```python
from build123d import *

# Parameters (mm, degrees)
CROQUIS1_W                       = 1396
CROQUIS1_H                       = 387.3
BRIDA_BASE1_DEPTH                = 3.175
TALADRO_DE_MARGEN_PARA_M51_D     = 5.5
BRIDA_DE_ARISTA1_STRIP_W         = 32.7
BRIDA_DE_ARISTA1_STRIP_H         = 3.175
BRIDA_DE_ARISTA1_STRIP_CUT_DEPTH = 1396
BRIDA_DE_ARISTA1_DEPTH           = 1396
TALADRO_DE_MARGEN_PARA_M52_D     = 5.5


# Sheet-metal steps are written as plain solids
with BuildPart() as part:
    # Croquis1 → Brida base1 (new body)
    with BuildSketch(Plane(origin=(0, 0, 0), x_dir=(1, 0, 0), z_dir=(0, 1, 0))):
        with Locations((-11.780590717, 234.868987342)):
            Rectangle(CROQUIS1_W, CROQUIS1_H)
    extrude(amount=-BRIDA_BASE1_DEPTH)

    # Taladro de margen para M51 (through all)
    with Locations(Plane(origin=(0, -3.175, 0), x_dir=(-1, 0, 0), z_dir=(0, -1, 0))):
        with Locations((508.430590717, 166.618987342), (508.430590717, 341.218987342), (308.430590717, 166.618987342), (308.430590717, 341.218987342), (108.430590717, 166.618987342), (108.430590717, 341.218987342), (-91.569409283, 166.618987342), (-91.569409283, 341.218987342), (-291.569409283, 166.618987342), (-291.569409283, 341.218987342), (-491.569409283, 166.618987342), (-491.569409283, 341.218987342), (667.430590717, 166.618987342), (667.430590717, 341.218987342), (-650.569409283, 166.618987342), (-650.569409283, 341.218987342)):
            Hole(TALADRO_DE_MARGEN_PARA_M51_D / 2)

    # Brida de arista1 strip (across the edge) → Brida de arista1 strip cut (cut)
    with BuildSketch(Plane(origin=(-709.780590717, -3.175, -428.518987342), x_dir=(0, 0, 1), z_dir=(1, 0, 0))):
        with Locations((-3.175, -1.5875)):
            Rectangle(BRIDA_DE_ARISTA1_STRIP_W, BRIDA_DE_ARISTA1_STRIP_H)
    extrude(amount=BRIDA_DE_ARISTA1_STRIP_CUT_DEPTH, mode=Mode.SUBTRACT)

    # Brida de arista1 section (across the edge) → Brida de arista1 (add)
    with BuildSketch(Plane(origin=(-709.780590717, -3.175, -428.518987342), x_dir=(0, 0, 1), z_dir=(1, 0, 0))):
        with BuildLine():
            Line((0, 10), (0, 296.825))
            Line((0, 296.825), (3.175, 296.825))
            Line((3.175, 296.825), (3.175, 10))
            ThreePointArc((3.175, 10), (6.103932188, 2.928932188), (13.175, 0))
            Line((13.175, 0), (13.175, -3.175))
            ThreePointArc((13.175, -3.175), (3.858868158, 0.683868158), (0, 10))
        make_face()
    extrude(amount=BRIDA_DE_ARISTA1_DEPTH)

    # Taladro de margen para M52 (through all)
    with Locations(Plane.XY.offset(-425.343987342)):
        with Locations((-687.930590717, -216.9), (-687.930590717, -38.2), (-487.930590717, -216.9), (-487.930590717, -38.2), (-287.930590717, -216.9), (-287.930590717, -38.2), (-128.930590717, -216.9), (-128.930590717, -38.2), (71.069409283, -216.9), (71.069409283, -38.2), (271.069409283, -216.9), (271.069409283, -38.2), (471.069409283, -216.9), (471.069409283, -38.2), (671.069409283, -216.9), (671.069409283, -38.2)):
            Hole(TALADRO_DE_MARGEN_PARA_M52_D / 2)


solid = part.part
```
Geometry: final body of the model. Coordinates: model frame, mm. A direction names the side the tool comes from. Give positions to 0.01 mm unless a question says otherwise; leave off trailing zeros. Loops run counter-clockwise (first coordinate to the right, second up) from the corner with the lowest first, then second, coordinate; pieces in that order, holes last. Notation, with made-up numbers: (71, -7) -> (80, -7) arc R20 cw to (80, 11) -> close; hole circle Ø4 at (-26, 87). An arc over 180 degrees is marked (long way). Use one line per item in the form item = value.
Item 1: Pin query (flat end, axial travel): P1, Ø5, axis at x = -508.43, z = -341.22, coming from the -Y side; P2, Ø1.5, axis at x = 470.5, z = -356.5, coming from the -Y side (3 decimals); P3, Ø2, axis at x = -84.5, y = -107, coming from the +Z side. Return the tip coordinate at first contact, or that it passes through.
A:
P1 = through
P2 = -3.175
P3 = -425.34
Item 2: Section query B-B on z = -196.5. Output: boundary loops of the cut face in (x, y) (3 decimals), and give its area (3 significant figures).
A:
outline = (-709.781, -3.175) -> (686.219, -3.175) -> (686.219, 0) -> (-709.781, 0) -> close
area = 4,430 mm^2
Item 3: Section query A-A on x = 455.5. Output: boundary loops of the cut face in (y, z) (3 decimals).
A:
outline = (-300, -428.519) -> (-13.175, -428.519) arc R13.175 ccw to (0, -415.344) -> (0, -41.219) -> (-3.175, -41.219) -> (-3.175, -415.344) arc R10 cw to (-13.175, -425.344) -> (-300, -425.344) -> close
Item 4: Access query for faces 1 (the face through (-22, 0, -231)), 2 (the face through (-22, -3.175, -231)). Directions: +Z, -Z, +X, -X, +Y, -Y. A direction counts if a zero-diameter tool reaches every point of the face in a straight line with its end or side. Return the directions, or none.
A:
face_1 = +Z, -Z, +X, -X, +Y
face_2 = +Z, +X, -X, -Y
Item 5: Line query: probe 1 along Y at (x, z) = (438.5, -109.5) (3 decimals); probe 2 along Z at (x, y) = (459, -51). Output: solid intervals per line, ascending.
A:
probe_1 = -3.175 to 0
probe_2 = -428.52 to -425.34
Item 6: Section query C-C on y = -102. Output: boundary loops of the cut face in (x, z).
A:
outline = (-709.78, -428.52) -> (686.22, -428.52) -> (686.22, -425.34) -> (-709.78, -425.34) -> close
